from build123d import *

# Parameters (mm, degrees)
BODY_DEPTH = 6
THREAD_R   = 3
HOLE_DEPTH = 10.712534856


with BuildPart() as part:
    # profile → body (new body)
    with BuildSketch(Plane(origin=(0, 0, 0), x_dir=(1, 0, 0), z_dir=(0, 1, 0))):
        Polygon((5.773502692, 0), (2.886751346, 5), (-2.886751346, 5), (-5.773502692, 0), (-2.886751346, -5), (2.886751346, -5), align=None)
    extrude(amount=BODY_DEPTH)

    # Sketch7 → fillet 2 (revolve, cut)
    with BuildSketch(Plane.XY):
        with BuildLine():
            Line((5.773502692, 5.23120945), (5.773502692, 0.76879055))
            ThreePointArc((5.773502692, 0.76879055), (2.974697147, -0.302787414), (0, -0.667161797))
            Line((0, -0.667161797), (0, -3.492163531))
            Line((0, -3.492163531), (6.272991846, -3.492163531))
            Line((6.272991846, -3.492163531), (6.272991846, 7.504587098))
            Line((6.272991846, 7.504587098), (0, 7.504587098))
            Line((0, 7.504587098), (0, 6.667161797))
            ThreePointArc((0, 6.667161797), (2.974697147, 6.302787414), (5.773502692, 5.23120945))
        make_face()
    revolve(axis=Axis((0, 0, 0), (0, 1, 0)), mode=Mode.SUBTRACT)

    # thread (on Top Plane) → hole (cut, through all)
    with BuildSketch(Plane(origin=(0, 0, 0), x_dir=(1, 0, 0), z_dir=(0, 1, 0))):
        with Locations(Location((0, 0, 0), (0, 0, 270))):
            Circle(THREAD_R)
    extrude(amount=HOLE_DEPTH, mode=Mode.SUBTRACT)


solid = part.part
Part model, mm, in its own coordinate system. Give positions to 0.01 mm unless a question says otherwise; leave off trailing zeros. Order: outer loops, then holes, each group sorted by start corner. A loop starts at its lowest first (then second) coordinate and runs counter-clockwise, first axis right, second up. Notation, with made-up numbers: (25, -21) - (53, -21) arc R18 ccw to (53, 2) - close; hole circle Ø9 at (6.25, -36.5). An arc over 180 degrees is marked (long way). Use a Markdown table: item, result.
1) Two-plate mould, pull along X, no slides. Class faces 1 (the flat face through (0, 3, -5)), 2 (the flat face through (-4.31, 2.963, -2.535)), 3 (the cylindrical face through (0.9, 2.96, 2.86)): +X half, -X half, draft (parallel to the pull), parting line (faces both ways), or undercut.
Checked values:
| item | result |
|---|---|
| face 1 | draft |
| face 2 | -X half |
| face 3 | undercut |
2) Saw through at C-C on y = 4.25. List the corners of the cut face in (x, z).
Checked values:
| item | result |
|---|---|
| outline | (-5.77, 0) - (-2.89, -5) - (2.89, -5) - (5.77, 0) - (2.89, 5) - (-2.89, 5) - close; hole circle Ø6 at (0, 0) |
3) Flat gauge pin, fed straight in: P1, Ø1, axis at x = 4, z = 3, coming from the +Y side. Where does the tip first touch, or does it go through?
Checked values:
| item | result |
|---|---|
| P1 | y = 5.82 |
4) Probe L1, parallel to Z at x = 0, y = 4.4; L2, parallel to Z at x = 1.5, y = 4.5; L3, parallel to X at y = 0.5, z = 0.25. List the from-to ranges inside material, lowest first. Write a range as from..to.
Checked values:
| item | result |
|---|---|
| L1 | -5..-3, 3..5 |
| L2 | -5..-2.6, 2.6..5 |
| L3 | -5.23..-2.99, 2.99..5.23 |
5) Saw through at D-D on z = 3.75. List the corners of the cut face in (x, y).
Checked values:
| item | result |
|---|---|
| outline | (-3.61, 0.49) arc R11.74 ccw to (-1.39, 0) - (1.39, 0) arc R11.74 ccw to (3.61, 0.49) - (3.61, 5.51) arc R11.74 ccw to (1.39, 6) - (-1.39, 6) arc R11.74 ccw to (-3.61, 5.51) - close |
6) Saw through at B-B on z = 1.5. List the corners of the cut face in (x, y).
Checked values:
| item | result |
|---|---|
| outline | (-4.91, 0.45) arc R12.23 ccw to (-3.71, 0) - (-2.6, 0) - (-2.6, 6) - (-3.71, 6) arc R12.23 ccw to (-4.91, 5.55) - close; (2.6, 0) - (3.71, 0) arc R12.23 ccw to (4.91, 0.45) - (4.91, 5.55) arc R12.23 ccw to (3.71, 6) - (2.6, 6) - close |
7) Saw through at A-A on x = 0. List the corners of the cut face in (y, z), plus the area to 3 significant figures.
Checked values:
| item | result |
|---|---|
| outline | (0, -4) arc R12.32 ccw to (0.39, -5) - (5.61, -5) arc R12.32 ccw to (6, -4) - (6, -3) - (0, -3) - close; (0, 3) - (6, 3) - (6, 4) arc R12.32 ccw to (5.61, 5) - (0.39, 5) arc R12.32 ccw to (0, 4) - close |
| area | 23.2 mm² |
